from build123d import *

# Parameters (mm, degrees)
EXTRUDE_1_DEPTH      = 15
EXTRUDE_1_DEPTH_BACK = 15
SKETCH_1_R           = 4
SKETCH_2_R           = 8
SKETCH_2_R_2         = 4
EXTRUDE_3_DEPTH      = 3
EXTRUDE_4_DEPTH      = 30
SKETCH_4_R           = 4
EXTRUDE_5_DEPTH      = 8
SKETCH_5_R           = 6
EXTRUDE_6_DEPTH      = 2
SKETCH_6_R           = 4
EXTRUDE_7_DEPTH      = 10


with BuildPart() as part:
    # 草图1 → 凸台-拉伸1 (new, two sides: drawn at the far end of the back side and taken through both)
    with BuildSketch(Plane(origin=(0, 0, 0), x_dir=(0, 0, -1), z_dir=(1, 0, 0)).offset(-EXTRUDE_1_DEPTH_BACK)):
        Circle(SKETCH_1_R)
    extrude(amount=EXTRUDE_1_DEPTH + EXTRUDE_1_DEPTH_BACK)

    # 草图2 → 凸台-拉伸3 (add)
    # profile 1 of 4: a face of its own
    with BuildSketch(Plane(origin=(15, 0, 0), x_dir=(0, 0, -1), z_dir=(1, 0, 0))):
        with Locations((-20, 40)):
            Circle(SKETCH_2_R)
    # profile 2 of 4: a face of its own
    with BuildSketch(Plane(origin=(15, 0, 0), x_dir=(0, 0, -1), z_dir=(1, 0, 0))):
        Circle(SKETCH_2_R)
        Circle(SKETCH_2_R_2, mode=Mode.SUBTRACT)
    # profile 3 of 4: a face of its own
    with BuildSketch(Plane(origin=(15, 0, 0), x_dir=(0, 0, -1), z_dir=(1, 0, 0))):
        Circle(SKETCH_2_R_2)
    # profile 4 of 4: a face of its own
    with BuildSketch(Plane(origin=(15, 0, 0), x_dir=(0, 0, -1), z_dir=(1, 0, 0))):
        with BuildLine():
            ThreePointArc((-12, 40), (-18.161976636, 32.214008084), (-27.155417528, 36.422291236))
            Line((-27.155417528, 36.422291236), (-7.155417528, -3.577708764))
            ThreePointArc((-7.155417528, -3.577708764), (-3.577708764, 7.155417528), (7.155417528, 3.577708764))
            Line((7.155417528, 3.577708764), (-12.844582472, 43.577708764))
            ThreePointArc((-12.844582472, 43.577708764), (-12.214008084, 41.838023364), (-12, 40))
        make_face()
    extrude_3 = extrude(amount=EXTRUDE_3_DEPTH)

    # 镜向2: 凸台-拉伸3 across plane
    add(extrude_3.mirror(Plane(origin=(0, 0, 0), x_dir=(0, 0, 1), z_dir=(1, 0, 0))))

    # 草图3 → 凸台-拉伸4 (add)
    with BuildSketch(Plane(origin=(-15, 0, 0), x_dir=(0, 0, -1), z_dir=(1, 0, 0))):
        with BuildLine():
            Line((-11.344582472, 40.577708764), (-12.844582472, 43.577708764))
            Line((-12.844582472, 43.577708764), (-27.155417528, 43.577708764))
            ThreePointArc((-27.155417528, 43.577708764), (-27.714499823, 42.118134198), (-27.979113521, 40.577708764))
            Line((-27.979113521, 40.577708764), (-11.344582472, 40.577708764))
        make_face()
    extrude(amount=EXTRUDE_4_DEPTH)

    # 草图4 → 凸台-拉伸5 (add)
    with BuildSketch(Plane(origin=(0, 43.577708764, 0), x_dir=(1, 0, 0), z_dir=(0, 1, 0))):
        with Locations(Location((0, -20, 0), (0, 0, 90))):
            Circle(SKETCH_4_R)
    extrude(amount=EXTRUDE_5_DEPTH)

    # 草图5 → 凸台-拉伸6 (add)
    with BuildSketch(Plane(origin=(0, 51.577708764, 0), x_dir=(1, 0, 0), z_dir=(0, 1, 0))):
        with Locations(Location((0, -20, 0), (0, 0, 270))):
            Circle(SKETCH_5_R)
    extrude(amount=EXTRUDE_6_DEPTH)

    # 草图6 → 凸台-拉伸7 (add)
    with BuildSketch(Plane(origin=(0, 53.577708764, 0), x_dir=(1, 0, 0), z_dir=(0, 1, 0))):
        with Locations(Location((0, -20, 0), (0, 0, 90))):
            Circle(SKETCH_6_R)
    extrude(amount=EXTRUDE_7_DEPTH)


solid = part.part
Geometry check sheet. Reference: the model listing, model coordinates, mm. A direction names the side the tool comes from. Give positions to 0.01 mm unless a question says otherwise; leave off trailing zeros. Write each loop counter-clockwise with the first axis right and the second up, starting at its lowest first coordinate (ties: lowest second). Pieces come first, ordered by that corner, then holes. Notation, with made-up numbers: M 52,10.5 L 103,10.5 A12 ccw 103,19.5 Z; hole C 82.25,19.25 d9. An arc over 180 degrees is marked long. One line per question, with ' | ' between items.
1. Scan lines: line 1 along X through (y, z) = (30, 10.5); line 2 along Y through (x, z) = (3, 13); line 3 along Y through (x, z) = (3, 18). Record each from-to range of solid material in increasing order. Write a range as from..to.
Ans:
line 1: -18..-15, 15..18 | line 2: 40.58..43.58 | line 3: 40.58..63.58
2. Set-up check for faces 1 (the face through (-0.21, -3.905, 0.867)), 2 (the face through (-2.3, 52.56, 25.54)), 3 (the face through (0, 40.578, 20)), 4 (the face through (15, 45, 20)): record each of +Z, -Z, +X, -X, +Y, -Y from which the full face is reachable in a straight line by a thin tool's end or side.
Ans:
face 1: none | face 2: +Y | face 3: +Z, -Z, -Y | face 4: +Z, -Z, +Y
3. Cross-section at D-D (x = 0). Enter the section's corners in (y, z).
Ans:
outline: C 0,0 d8; M 40.58,11.34 L 43.58,12.84 L 43.58,16 L 51.58,16 L 51.58,14 L 53.58,14 L 53.58,16 L 63.58,16 L 63.58,24 L 53.58,24 L 53.58,26 L 51.58,26 L 51.58,24 L 43.58,24 L 43.58,27.16 A8 ccw 40.58,27.98 Z
4. Cross-section at B-B (x = -9). Enter the section's corners in (y, z), plus the area to 3 significant figures.
Ans:
outline: C 0,0 d8; M 40.58,11.34 L 43.58,12.84 L 43.58,27.16 A8 ccw 40.58,27.98 Z | area: 97.0 mm2
5. Mould release check, pull along Y, two halves, no side actions. Record for faces 5 (the face through (18, 20, 10)), 6 (the face through (16.48, -7.23, -3.42)), 7 (the face through (0, 63.578, 20)), 8 (the face through (2.4, 47.5, 23.2)): released by +Y, released by -Y, zero draft, split by the parting line, or undercut.
Ans:
face 5: zero draft | face 6: split by the parting line | face 7: released by +Y | face 8: undercut
6. Cross-section at A-A (y = 37.5). Enter the section's corners in (x, z), plus the area to 3 significant figures.
Ans:
outline: M -18,9.81 L -15,9.81 L -15,27.6 L -18,27.6 Z; M 15,9.81 L 18,9.81 L 18,27.6 L 15,27.6 Z | area: 107 mm2
7. Cross-section at C-C (z = 0). Enter the section's corners in (x, y).
Ans:
outline: M -18,-8 L -15,-8 L -15,-4 L 15,-4 L 15,-8 L 18,-8 L 18,17.89 L 15,17.89 L 15,4 L -15,4 L -15,17.89 L -18,17.89 Z
8. Gauge pin test, flat ends, axial feed: pin 1 (1 mm diameter, centred on y = 51, z = 21, fed in from +X); pin 2 (4 mm diameter, centred on x = 12, z = 23.5, fed in from -Y); pin 3 (4 mm diameter, centred on x = -1.5, y = 1, fed in from -Z). Record the tip position at first contact, or that the pin passes through.
Ans:
pin 1: x = 3.97 | pin 2: y = 40.58 | pin 3: z = -4
